The drawing under review shows one solid part. Ordinate dimensions are in mm from its lowest x, y, z. A direction names the side the tool comes from. Coordinates: 2 decimals unless noted, no trailing zeros. Write each loop counter-clockwise with the first axis right and the second up, starting at its lowest first coordinate (ties: lowest second). Pieces come first, ordered by that corner, then holes.
1) For line 1 (Y direction, x = 366.5, z = 112.5); line 2 (X direction, y = 389.25, z = 140); line 3 (Y direction, x = 324, z = 7), list the stretches that pass through material, from the lowest coordinate up.
2) Add section D-D, the plane z = 140. State the section outline as (x, y) points, then the cut area to 3 significant figures.
3) Add section B-B, the plane y = 76. State the section outline as (x, z) points, then the cut area to 3 significant figures.
4) Add section C-C, the plane z = 170.5. State the section outline as (x, y) points, then the cut area to 3 significant figures.
5) Mouldability with a two-part tool opening along X and no side actions: class the marked faces 3, 4, 5 and 6 as released by +X, released by -X, zero draft, split by the parting line, or undercut.
6) For P1, Ø1.5, axis at x = 351.5, y = 73, coming from the +Z side, flat-tipped, find the tip position at first contact; note if it passes through.
7) Machinability: for the marked faces 1 and 2, which of the approach directions +Z, -Z, +X, -X, +Y, -Y give a long, thin tool a straight path to every point of the face, cutting with its end or side? Answer none if there is none.
8) Add section A-A, the plane x = 339. State the section outline as (y, z) points, then the cut area to 3 significant figures.
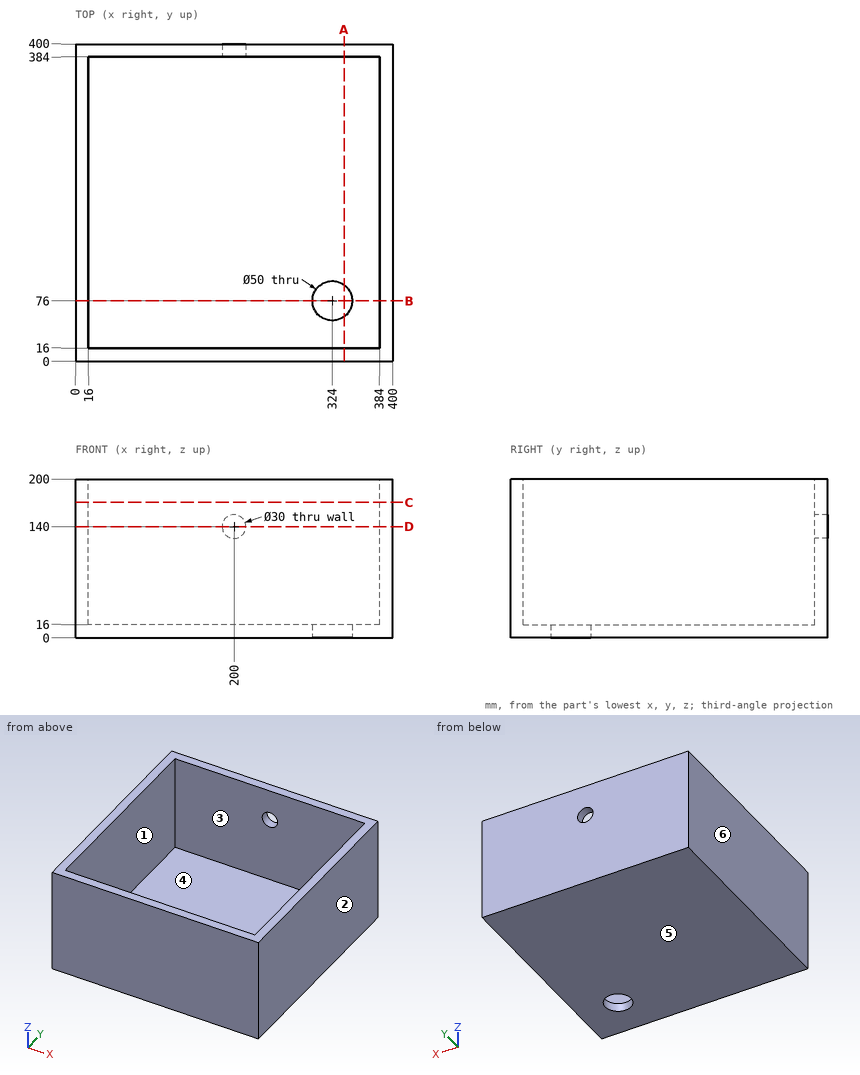
Geometry results:
1. line 1: y = 0 to 16, 384 to 400
1. line 2: x = 0 to 185, 215 to 400
1. line 3: y = 0 to 51, 101 to 400
2. outline: (0, 0) - (400, 0) - (400, 400) - (215, 400) - (215, 384) - (384, 384) - (384, 16) - (16, 16) - (16, 384) - (185, 384) - (185, 400) - (0, 400) - close
2. area: 24,100 mm2
3. outline: (0, 0) - (299, 0) - (299, 16) - (16, 16) - (16, 200) - (0, 200) - close; (349, 0) - (400, 0) - (400, 200) - (384, 200) - (384, 16) - (349, 16) - close
3. area: 11,500 mm2
4. outline: (0, 0) - (400, 0) - (400, 400) - (0, 400) - close; hole (16, 16) - (384, 16) - (384, 384) - (16, 384) - close
4. area: 24,600 mm2
5. face 3: undercut
5. face 4: undercut
5. face 5: zero draft
5. face 6: released by -X
6. P1: stops at z = 16
7. face 1: +Z
7. face 2: +Z, -Z, +X, +Y, -Y
8. outline: (0, 0) - (56, 0) - (56, 16) - (16, 16) - (16, 200) - (0, 200) - close; (96, 0) - (400, 0) - (400, 200) - (384, 200) - (384, 16) - (96, 16) - close
8. area: 11,600 mm2
